Read the model definition and answer for the solid it produces. Units are mm, in the model's axes. A direction names the side the tool comes from. Coordinates: 2 decimals unless noted, no trailing zeros. Loops run counter-clockwise (first coordinate to the right, second up) from the corner with the lowest first, then second, coordinate; pieces in that order, holes last. Notation, with made-up numbers: (78.5, 11) -> (136.5, 11) arc R20 ccw to (136.5, 37) -> close; hole circle Ø1 at (-37, 21.5). An arc over 180 degrees is marked (long way). Answer as a JSON object with one key per item and string values. Group by question number.
1) Section B-B, the plane y = 7.5 is taken. Give the vertices of the cut face in (x, z) (1 decimal), plus the area to 3 significant figures.
2) Which of the six approach directions +Z, -Z, +X, -X, +Y, -Y give full straight-line access (tool end or side, diameter ignored) to faces 1 (the face through (-18.22, -25.72, -77.83)), 2 (the face through (2.58, -22.23, -74.2)), 3 (the face through (-20, 25.146, -1))?
3) Section C-C, the plane z = 18 is taken. Give the vertices of the cut face in (x, y) (1 decimal), plus the area to 3 significant figures.
4) Flat-ended cylindrical pins translate along their axes: P1, Ø3, axis at y = 4, z = 28, coming from the -X side; P2, Ø1.5, axis at y = 0, z = 55.5, coming from the +X side. Find the tip coordinate at first contact, or state that the pin passes through.
5) Consider probe 1 along Z at (x, y) = (-4.5, -10); probe 2 along Y at (x, z) = (-19, 32); probe 3 along X at (y, z) = (2, 31). Determine where each line is inside the solid, lowest interval first. Write a range as [from, to].
from build123d import *

# Parameters (mm, degrees)
F1_DEPTH = 1.524
F3_DEPTH = 40.132
F5_DEPTH = 2.794
F8_R     = 1.5875
F9_R     = 1.5875
F10_R    = 1.5875
F11_R    = 1.5875


with BuildPart() as f1:
    # F0 (on Right) → F1 (new body)
    with BuildSketch(Plane.YZ):
        with BuildLine():
            ThreePointArc((26.67, 75.565), (25.7400640303, 77.8100640303), (23.495, 78.74))
            Line((23.495, 78.74), (-23.495, 78.74))
            ThreePointArc((-23.495, 78.74), (-25.7400640303, 77.8100640303), (-26.67, 75.565))
            Line((-26.67, 75.565), (-26.67, -75.565))
            ThreePointArc((-26.67, -75.565), (-25.7400640303, -77.8100640303), (-23.495, -78.74))
            Line((-23.495, -78.74), (23.495, -78.74))
            ThreePointArc((23.495, -78.74), (25.7400640303, -77.8100640303), (26.67, -75.565))
            Line((26.67, -75.565), (26.67, 75.565))
        make_face()
    extrude(amount=F1_DEPTH)

    # F2 (on face) → F3 (join)
    with BuildSketch(Plane(origin=(0, 0, 0), x_dir=(0, -1, 0), z_dir=(-1, 0, 0))):
        with BuildLine():
            Line((23.495, 78.74), (-23.495, 78.74))
            ThreePointArc((-23.495, 78.74), (-25.7400640303, 77.8100640303), (-26.67, 75.565))
            Line((-26.67, 75.565), (-26.67, -75.565))
            ThreePointArc((-26.67, -75.565), (-25.7400640303, -77.8100640303), (-23.495, -78.74))
            Line((-23.495, -78.74), (23.495, -78.74))
            ThreePointArc((23.495, -78.74), (25.7400640303, -77.8100640303), (26.67, -75.565))
            Line((26.67, -75.565), (26.67, 75.565))
            ThreePointArc((26.67, 75.565), (25.7400640303, 77.8100640303), (23.495, 78.74))
        make_face()
        with BuildLine():
            ThreePointArc((25.146, -75.6285), (24.6810320151, -76.7510320151), (23.5585, -77.216))
            Line((23.5585, -77.216), (-23.5585, -77.216))
            ThreePointArc((-23.5585, -77.216), (-24.6810320151, -76.7510320151), (-25.146, -75.6285))
            Line((-25.146, -75.6285), (-25.146, 75.6285))
            ThreePointArc((-25.146, 75.6285), (-24.6810320151, 76.7510320151), (-23.5585, 77.216))
            Line((-23.5585, 77.216), (23.5585, 77.216))
            ThreePointArc((23.5585, 77.216), (24.6810320151, 76.7510320151), (25.146, 75.6285))
            Line((25.146, 75.6285), (25.146, -75.6285))
        make_face(mode=Mode.SUBTRACT)
    extrude(amount=F3_DEPTH)

    # F4 (on face) → F5 (join)
    with BuildSketch(Plane.YZ.offset(1.524)):
        with BuildLine():
            ThreePointArc((-26.67, 72.39), (-22.1798719395, 74.2498719395), (-20.32, 78.74))
            Line((-20.32, 78.74), (-23.495, 78.74))
            ThreePointArc((-23.495, 78.74), (-25.7400640303, 77.8100640303), (-26.67, 75.565))
            Line((-26.67, 75.565), (-26.67, 72.39))
        make_face()
    extrude(amount=F5_DEPTH)


with BuildPart() as f6_1:
    # F6: instance of F1
    add(f1.part.mirror(Plane.XY))


with BuildPart() as f1_1:
    add(f1.part)

    add(f6_1.part)  # F7 merges F6_1
    # F7: F6_1, F1 across plane
    add(f6_1.part.mirror(Plane.XZ))
    add(f1.part.mirror(Plane.XZ))

    # F8
    f8_edges = [f1_1.edges().sort_by_distance(p)[0] for p in [
        (1.524, -26.67, 0),
    ]]
    fillet(f8_edges, radius=F8_R)

    # F9
    f9_edges = [f1_1.edges().sort_by_distance(p)[0] for p in [
        (1.524, 0, -78.74),
    ]]
    fillet(f9_edges, radius=F9_R)

    # F10
    f10_edges = [f1_1.edges().sort_by_distance(p)[0] for p in [
        (1.524, 26.67, 0),
    ]]
    fillet(f10_edges, radius=F10_R)

    # F11
    f11_edges = [f1_1.edges().sort_by_distance(p)[0] for p in [
        (1.524, 0, 78.74),
    ]]
    fillet(f11_edges, radius=F11_R)


solid = f1_1.part
Determined:
{
 "1": {"outline": "(-40.1, -78.7) -> (-0.1, -78.7) arc R1.6 ccw to (1.5, -77.2) -> (1.5, 77.2) arc R1.6 ccw to (-0.1, 78.7) -> (-40.1, 78.7) -> (-40.1, 77.2) -> (0, 77.2) -> (0, -77.2) -> (-40.1, -77.2) -> close", "area": "361 mm²"},
 "2": {"face 1": "-Z, +X, -X, -Y", "face 2": "+X", "face 3": "-X"},
 "3": {"outline": "(-40.1, -26.7) -> (-0.1, -26.7) arc R1.6 ccw to (1.5, -25.1) -> (1.5, 25.1) arc R1.6 ccw to (-0.1, 26.7) -> (-40.1, 26.7) -> (-40.1, 25.1) -> (0, 25.1) -> (0, -25.1) -> (-40.1, -25.1) -> close", "area": "203 mm²"},
 "4": {"P1": "x = 0", "P2": "x = 1.52"},
 "5": {"probe 1": "[-78.74, -77.22], [77.22, 78.74]", "probe 2": "[-26.67, -25.15], [25.15, 26.67]", "probe 3": "[0, 1.52]"}
}
